For this review, take the finished solid that the model builds, in its own axes (mm). Coordinates: 2 decimals unless noted, no trailing zeros. Loops run counter-clockwise (first coordinate to the right, second up) from the corner with the lowest first, then second, coordinate; pieces in that order, holes last. Notation, with made-up numbers: (80.25, 19) -> (135.25, 19) arc R15 ccw to (135.25, 33) -> close; hole circle Ø1 at (20.5, 32.25). An arc over 180 degrees is marked (long way). Use a Markdown table: item, result.
from build123d import *

# Parameters (mm, degrees)
CROQUIS1_R              = 2
CROQUIS1_R_2            = 4.5
CROQUIS1_R_3            = 6.198274882
CROQUIS1_R_4            = 1.5
CROQUIS1_R_5            = 9.306378824
SALIENTE_EXTRUIR1_DEPTH = 2


with BuildPart() as part:
    # Croquis1 → Saliente-Extruir1 (new body)
    with BuildSketch(Plane.XY):
        with BuildLine():
            Line((2814.976573627, 1239.042814145), (2832.341923679, 1239.042814145))
            ThreePointArc((2832.341923679, 1239.042814145), (2832.901941116, 1239.011353213), (2833.454911085, 1238.917366333))
            ThreePointArc((2833.454911085, 1238.917366333), (2888.36527428, 1232.640523344), (2943.314155481, 1238.570717173))
            ThreePointArc((2943.314155481, 1238.570717173), (2943.852021738, 1238.659519694), (2944.396358769, 1238.689238294))
            Line((2944.396358769, 1238.689238294), (2989.714258788, 1238.689238294))
            ThreePointArc((2989.714258788, 1238.689238294), (3007.214258788, 1221.189238294), (2989.714258788, 1203.689238294))
            Line((2989.714258788, 1203.689238294), (2943.987436651, 1203.689238294))
            ThreePointArc((2943.987436651, 1203.689238294), (2943.452657793, 1203.717919397), (2942.924014155, 1203.803633664))
            ThreePointArc((2942.924014155, 1203.803633664), (2888.146718467, 1209.523748699), (2833.444892603, 1203.122023463))
            ThreePointArc((2833.444892603, 1203.122023463), (2832.886438978, 1203.026115147), (2832.320719962, 1202.994008262))
            Line((2832.320719962, 1202.994008262), (2814.976573627, 1202.994008262))
            ThreePointArc((2814.976573627, 1202.994008262), (2812.148146502, 1204.165581137), (2810.976573627, 1206.994008262))
            Line((2810.976573627, 1206.994008262), (2810.976573627, 1235.042814145))
            ThreePointArc((2810.976573627, 1235.042814145), (2812.148146502, 1237.871241269), (2814.976573627, 1239.042814145))
        make_face()
        with Locations((2819.024210059, 1231.146271353)):
            Circle(CROQUIS1_R, mode=Mode.SUBTRACT)
        with Locations((2989.714258788, 1221.189238294)):
            Circle(CROQUIS1_R_2, mode=Mode.SUBTRACT)
        with Locations((2819.05924577, 1210.890776447)):
            Circle(CROQUIS1_R, mode=Mode.SUBTRACT)
        with Locations((2831.917693785, 1221.023549437)):
            Circle(CROQUIS1_R_3, mode=Mode.SUBTRACT)
        with Locations((2847.093240202, 1221.039483998)):
            Circle(CROQUIS1_R_3, mode=Mode.SUBTRACT)
        with Locations((2862.26878662, 1221.055418559)):
            Circle(CROQUIS1_R_3, mode=Mode.SUBTRACT)
        with Locations((2966.996257677, 1221.189238294)):
            Circle(CROQUIS1_R_4, mode=Mode.SUBTRACT)
        with Locations((2976.996257677, 1221.189238294)):
            Circle(CROQUIS1_R_4, mode=Mode.SUBTRACT)
        with Locations((2955.642950592, 1221.189238294)):
            Circle(CROQUIS1_R, mode=Mode.SUBTRACT)
        with Locations((2935.388208278, 1221.189238294)):
            Circle(CROQUIS1_R_5, mode=Mode.SUBTRACT)
        with Locations((2897.973392618, 1221.039483998)):
            Circle(CROQUIS1_R_3, mode=Mode.SUBTRACT)
        with Locations((2913.148939036, 1221.055418559)):
            Circle(CROQUIS1_R_3, mode=Mode.SUBTRACT)
        with BuildLine():
            Line((2982.289637586, 1215.885937435), (2980.168317242, 1213.764617091))
            ThreePointArc((2980.168317242, 1213.764617091), (2980.168317242, 1211.643296748), (2982.289637586, 1211.643296748))
            Line((2982.289637586, 1211.643296748), (2984.410957929, 1213.764617091))
            ThreePointArc((2984.410957929, 1213.764617091), (2984.410957929, 1215.885937435), (2982.289637586, 1215.885937435))
        make_face(mode=Mode.SUBTRACT)
        with BuildLine():
            Line((2995.017559647, 1213.764617091), (2997.138879991, 1211.643296748))
            ThreePointArc((2997.138879991, 1211.643296748), (2999.260200334, 1211.643296748), (2999.260200334, 1213.764617091))
            Line((2999.260200334, 1213.764617091), (2997.138879991, 1215.885937435))
            ThreePointArc((2997.138879991, 1215.885937435), (2995.017559647, 1215.885937435), (2995.017559647, 1213.764617091))
        make_face(mode=Mode.SUBTRACT)
        with BuildLine():
            Line((2997.138879991, 1226.492539153), (2999.260200334, 1228.613859496))
            ThreePointArc((2999.260200334, 1228.613859496), (2999.260200334, 1230.73517984), (2997.138879991, 1230.73517984))
            Line((2997.138879991, 1230.73517984), (2995.017559647, 1228.613859496))
            ThreePointArc((2995.017559647, 1228.613859496), (2995.017559647, 1226.492539153), (2997.138879991, 1226.492539153))
        make_face(mode=Mode.SUBTRACT)
        with BuildLine():
            Line((2984.410957929, 1228.613859496), (2982.289637586, 1230.73517984))
            ThreePointArc((2982.289637586, 1230.73517984), (2980.168317242, 1230.73517984), (2980.168317242, 1228.613859496))
            Line((2980.168317242, 1228.613859496), (2982.289637586, 1226.492539153))
            ThreePointArc((2982.289637586, 1226.492539153), (2984.410957929, 1226.492539153), (2984.410957929, 1228.613859496))
        make_face(mode=Mode.SUBTRACT)
        with BuildLine():
            Line((2950.185413449, 1233.422506858), (2972.422006236, 1233.422506858))
            ThreePointArc((2972.422006236, 1233.422506858), (2974.922006236, 1230.922506858), (2972.422006236, 1228.422506858))
            Line((2972.422006236, 1228.422506858), (2950.185413449, 1228.422506858))
            ThreePointArc((2950.185413449, 1228.422506858), (2947.685413449, 1230.922506858), (2950.185413449, 1233.422506858))
        make_face(mode=Mode.SUBTRACT)
        with BuildLine():
            Line((2950.185413449, 1208.955969729), (2972.422006236, 1208.955969729))
            ThreePointArc((2972.422006236, 1208.955969729), (2974.922006236, 1211.455969729), (2972.422006236, 1213.955969729))
            Line((2972.422006236, 1213.955969729), (2950.185413449, 1213.955969729))
            ThreePointArc((2950.185413449, 1213.955969729), (2947.685413449, 1211.455969729), (2950.185413449, 1208.955969729))
        make_face(mode=Mode.SUBTRACT)
    extrude(amount=SALIENTE_EXTRUIR1_DEPTH)


solid = part.part
(1) Take a section at A-A on x = 2845.5. Write out the cut boundary in (y, z).
Found:
| item | result |
|---|---|
| outline | (1205.59, 0) -> (1215.05, 0) -> (1215.05, 2) -> (1205.59, 2) -> close; (1227.03, 0) -> (1236.48, 0) -> (1236.48, 2) -> (1227.03, 2) -> close |
(2) For line 1 along Y through (x, z) = (2972, 0.45); line 2 along X through (y, z) = (1213, 1.75); line 3 along Y through (x, z) = (2981.5, 1.8), list the stretches that pass through material, from the lowest coordinate up.
Found:
| item | result |
|---|---|
| line 1 | y = 1203.69 to 1208.96, 1213.96 to 1228.42, 1233.42 to 1238.69 |
| line 2 | x = 2810.98 to 2930.97, 2939.81 to 2948.22, 2974.39 to 2979.76, 2983.65 to 2995.78, 2999.67 to 3005.18 |
| line 3 | y = 1203.69 to 1211.23, 1215.1 to 1227.28, 1231.15 to 1238.69 |
(3) Take a section at D-D on x = 2885.5. Write out the cut boundary in (y, z), plus the area to 3 significant figures.
Found:
| item | result |
|---|---|
| outline | (1209.49, 0) -> (1232.67, 0) -> (1232.67, 2) -> (1209.49, 2) -> close |
| area | 46.3 mm^2 |
(4) For pin 1 Ø15 at (x, y) = (2935.39, 1221.19) entering from -Z; pin 2 Ø1 at (y, z) = (1231.5, 1) entering from +X; pin 3 Ø0.6 at (x, z) = (2961, 1) entering from -Y, all flat-tipped, find the tip position at first contact; note any pin that passes through.
Found:
| item | result |
|---|---|
| pin 1 | passes through |
| pin 2 | stops at x = 3004.21 |
| pin 3 | stops at y = 1203.69 |
(5) Take a section at C-C on x = 2916. Write out the cut boundary in (y, z), plus the area to 3 significant figures.
Found:
| item | result |
|---|---|
| outline | (1208.14, 0) -> (1215.55, 0) -> (1215.55, 2) -> (1208.14, 2) -> close; (1226.56, 0) -> (1234.08, 0) -> (1234.08, 2) -> (1226.56, 2) -> close |
| area | 29.9 mm^2 |
(6) Mouldability with a two-part tool opening along X and no side actions: class faces 1 (the face through (2910, 1229, 0)), 2 (the face through (2868, 1218.7, 1)), 3 (the face through (2812.179, 1204.135, 0.986)), 4 (the face through (2916.009, 1215.556, 0.986)) as pulls with the +X half, pulls with the -X half, needs draft (parallel to the pull), parting line crosses it, or undercut.
Found:
| item | result |
|---|---|
| face 1 | needs draft |
| face 2 | undercut |
| face 3 | pulls with the -X half |
| face 4 | undercut |
(7) Take a section at B-B on z = 1.5. State how many separate pieces and enclosed holes the cut face has, plus the area to 3 significant figures.
Found:
| item | result |
|---|---|
| separate pieces | 1 |
| enclosed holes | 18 |
| area | 4,580 mm^2 |
